from build123d import *

# Parameters (mm, degrees)
AUFSATZ_LINEAR_AUSTRAGEN3_DEPTH      = 80
SCHNITT_LINEAR_AUSTRAGEN1_DEPTH      = 150.666295471
SCHNITT_LINEAR_AUSTRAGEN1_DEPTH_BACK = 150.666295471
SKIZZE10_R                           = 5.25
SCHNITT_LINEAR_AUSTRAGEN2_DEPTH      = 108.703296143
SCHNITT_LINEAR_AUSTRAGEN2_DEPTH_BACK = 108.703296143
AUFSATZ_LINEAR_AUSTRAGEN4_DEPTH      = 45
LINEARES_MUSTER1_COUNT               = 7
LINEARES_MUSTER1_PITCH               = 6
SKIZZE19_W                           = 160
SKIZZE19_H                           = 35
SCHNITT_LINEAR_AUSTRAGEN3_DEPTH      = 32


with BuildPart() as part:
    # Skizze9 → Aufsatz-Linear austragen3 (new, symmetric)
    with BuildSketch(Plane(origin=(0, 0, 0), x_dir=(0, 0, -1), z_dir=(1, 0, 0))):
        Polygon((-60, 40), (-60, 0), (60, 0), (60, 40), (55, 40), (55, 5), (-55, 5), (-55, 40), align=None)
    extrude(amount=AUFSATZ_LINEAR_AUSTRAGEN3_DEPTH, both=True)

    # Skizze10 → Schnitt-Linear austragen1 (cut, two sides: drawn at the far end of the back side and taken through both)
    with BuildSketch(Plane.XY.offset(60).offset(-SCHNITT_LINEAR_AUSTRAGEN1_DEPTH_BACK)):
        with Locations(Location((-69.5, 29.5, 0), (0, 0, 270))):
            Circle(SKIZZE10_R)
        with BuildLine():
            Line((25, 34.75), (72, 34.75))
            ThreePointArc((72, 34.75), (77.25, 29.5), (72, 24.25))
            Line((72, 24.25), (25, 24.25))
            ThreePointArc((25, 24.25), (19.75, 29.5), (25, 34.75))
        make_face()
    extrude(amount=SCHNITT_LINEAR_AUSTRAGEN1_DEPTH + SCHNITT_LINEAR_AUSTRAGEN1_DEPTH_BACK, mode=Mode.SUBTRACT)

    # Skizze12 → Schnitt-Linear austragen2 (cut, two sides: drawn at the far end of the back side and taken through both)
    with BuildSketch(Plane.XY.offset(-SCHNITT_LINEAR_AUSTRAGEN2_DEPTH_BACK)):
        with BuildLine():
            Line((-4, 40), (4, 40))
            ThreePointArc((4, 40), (0, 36), (-4, 40))
        make_face()
    extrude(amount=SCHNITT_LINEAR_AUSTRAGEN2_DEPTH + SCHNITT_LINEAR_AUSTRAGEN2_DEPTH_BACK, mode=Mode.SUBTRACT)

    # Skizze18 → Aufsatz-Linear austragen4 (add)
    with BuildSketch(Plane(origin=(0, 0, 0), x_dir=(-1, 0, 0), z_dir=(0, 0, -1))):
        with BuildLine():
            Line((-32, 5), (-38, 5))
            add(Edge.make_bspline(
                [(-38, 5), (-35.16767955, 7.124664511), (-32, 7)],
                knots=[0, 0, 0, 0.477297659, 0.477297659, 0.477297659], degree=2))
            Line((-32, 7), (-32, 5))
        make_face()
    aufsatz_linear_austragen4 = extrude(amount=-AUFSATZ_LINEAR_AUSTRAGEN4_DEPTH)

    # Lineares Muster1: Aufsatz-Linear austragen4 ×7
    with Locations(*[(i * LINEARES_MUSTER1_PITCH, 0, 0) for i in range(1, LINEARES_MUSTER1_COUNT)]):
        add(aufsatz_linear_austragen4)

    # Skizze19 → Schnitt-Linear austragen3 (cut)
    with BuildSketch(Plane.XY):
        with Locations((0, 22.5)):
            Rectangle(SKIZZE19_W, SKIZZE19_H)
    extrude(amount=SCHNITT_LINEAR_AUSTRAGEN3_DEPTH, mode=Mode.SUBTRACT)


solid = part.part
Could you check a few things on this model? Use its own coordinates, in mm. A direction names the side the tool comes from. Give positions to 0.01 mm unless a question says otherwise; leave off trailing zeros. Order: outer loops, then holes, each group sorted by start corner. A loop starts at its lowest first (then second) coordinate and runs counter-clockwise, first axis right, second up. Notation, with made-up numbers: (-33, 26.25) - (-14, 26.25) arc R22 cw to (-14, 52.25) - close; hole circle Ø8 at (57.25, -36.75). An arc over 180 degrees is marked (long way). One line per item, written item: value. Start each with the question number.
1. Imagine slicing it at D-D on x = 0. List the corners of the cut face in (y, z) for me, plus the area to 3 significant figures.
2. If I drill on probe 1 along X at (y, z) = (29.5, -58.9); probe 2 along Z at (x, y) = (-6.5, 27); probe 3 along Y at (x, z) = (-69.5, 56.45), over which ranges is the centre line in solid material (lowest first)?
3. For faces 1 (the face through (-41, 40, -58)), 2 (the face through (19.75, 29.38, 57.46)), 3 (the face through (1, 22, 55)), which set-ups out of +Z, -Z, +X, -X, +Y, -Y let a thin tool reach every point of the face, with its end or its side?
4. Imagine slicing it at C-C on z = 50. List the corners of the cut face in (x, y) for me.
5. For P1, Ø3, axis at x = 22.5, z = -4, coming from the +Y side; P2, Ø1, axis at y = 6.5, z = 41, coming from the -X side, each with a flat end and sliding along its axis, tell me the tip position at first contact or that it passes through.
6. Thinking about a two-plate mould opening in X: for faces 4 (the face through (80, 2, 0)), 5 (the face through (-1, 5, -1)), 6 (the face through (-74.625, 30.638, 57.465)), which applies, +X half, -X half, draft (parallel to the pull), parting line (faces both ways), or undercut?
7. Imagine slicing it at A-A on x = -69.5. List the corners of the cut face in (y, z) for me, plus the area to 3 significant figures.
8. Imagine slicing it at B-B on x = -49.5. List the corners of the cut face in (y, z) for me.
Values:
1. outline: (0, -60) - (36, -60) - (36, -55) - (5, -55) - (5, 55) - (36, 55) - (36, 60) - (0, 60) - close
1. area: 910 mm²
2. probe 1: -80 to -74.75, -64.25 to 19.75, 77.25 to 80
2. probe 2: -60 to -55, 55 to 60
2. probe 3: 0 to 24.25, 34.75 to 40
3. face 1: +Z, -Z, +X, -X, +Y
3. face 2: +Z, -Z
3. face 3: +X, -X, +Y
4. outline: (-80, 0) - (80, 0) - (80, 5) - (-80, 5) - close
5. P1: y = 5
5. P2: x = 32
6. face 4: +X half
6. face 5: draft
6. face 6: undercut
7. outline: (0, -60) - (24.25, -60) - (24.25, -55) - (5, -55) - (5, 55) - (24.25, 55) - (24.25, 60) - (0, 60) - close; (34.75, -60) - (40, -60) - (40, -55) - (34.75, -55) - close; (34.75, 55) - (40, 55) - (40, 60) - (34.75, 60) - close
7. area: 845 mm²
8. outline: (0, -60) - (40, -60) - (40, -55) - (5, -55) - (5, 55) - (40, 55) - (40, 60) - (0, 60) - close
